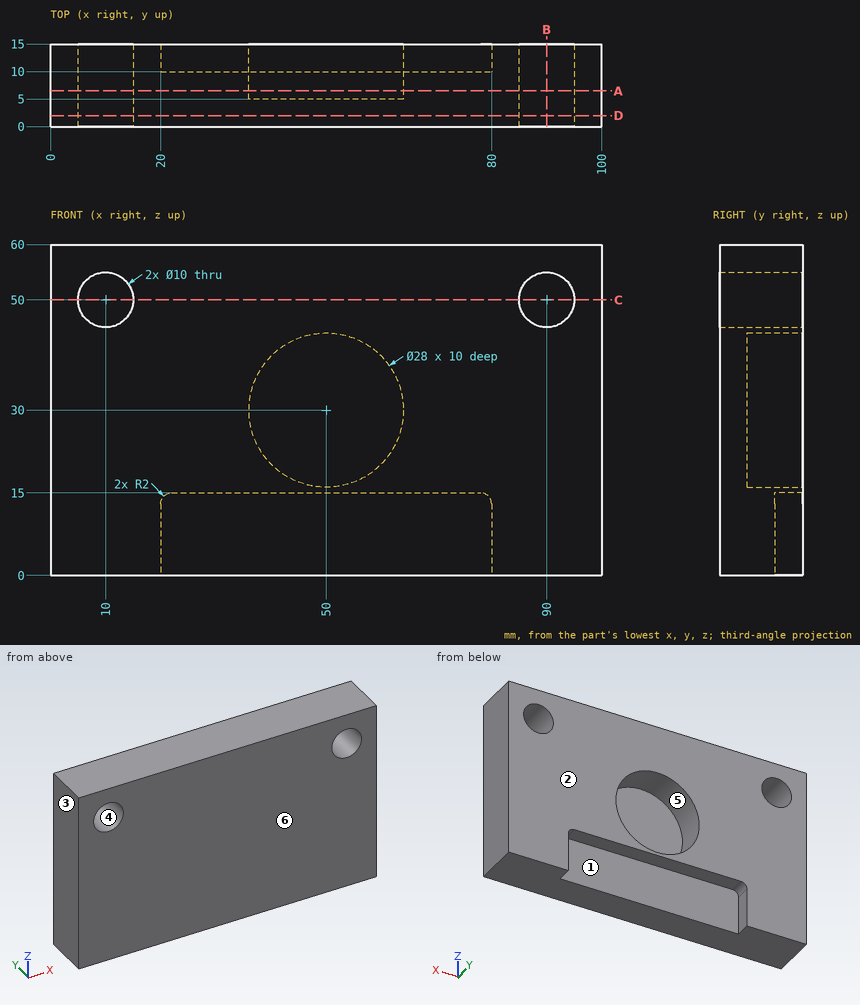
The drawing under review shows one solid part. Ordinate dimensions are in mm from its lowest x, y, z. A direction names the side the tool comes from. Coordinates: 2 decimals unless noted, no trailing zeros. Loops run counter-clockwise (first coordinate to the right, second up) from the corner with the lowest first, then second, coordinate; pieces in that order, holes last. Notation, with made-up numbers: (37, -39.75) -> (83, -39.75) arc R17 cw to (83, -26.75) -> close; hole circle Ø1 at (71.25, 81.25). An arc over 180 degrees is marked (long way). Answer as a JSON object with one key per item and string values.
Q1. Take a section at A-A on y = 6.5. Give the boundary of the cut face in (x, z), plus the area to 3 significant figures.
Answer block:
{"outline": "(0, 0) -> (100, 0) -> (100, 60) -> (0, 60) -> close; hole circle Ø10 at (10, 50); hole circle Ø28 at (50, 30); hole circle Ø10 at (90, 50)", "area": "5,230 mm^2"}
Q2. Take a section at D-D on y = 2. Give the boundary of the cut face in (x, z), plus the area to 3 significant figures.
Answer block:
{"outline": "(0, 0) -> (100, 0) -> (100, 60) -> (0, 60) -> close; hole circle Ø10 at (10, 50); hole circle Ø10 at (90, 50)", "area": "5,840 mm^2"}
Q3. Take a section at C-C on z = 50. Give the boundary of the cut face in (x, y).
Answer block:
{"outline": "(0, 0) -> (5, 0) -> (5, 15) -> (0, 15) -> close; (15, 0) -> (85, 0) -> (85, 15) -> (15, 15) -> close; (95, 0) -> (100, 0) -> (100, 15) -> (95, 15) -> close"}
Q4. Tool access review of the marked faces 5 and 6: name each direction out of +Z, -Z, +X, -X, +Y, -Y from which nothing blocks a thin tool from reaching the whole face with its end or side.
Answer block:
{"face 5": "+Y", "face 6": "+Z, -Z, +X, -X, -Y"}
Q5. Take a section at B-B on x = 90. Give the boundary of the cut face in (y, z), plus the area to 3 significant figures.
Answer block:
{"outline": "(0, 0) -> (15, 0) -> (15, 45) -> (0, 45) -> close; (0, 55) -> (15, 55) -> (15, 60) -> (0, 60) -> close", "area": "750 mm^2"}
Q6. Clearance check with flat-ended pins moving along their axes: pin 1 Ø7.5 at (x, z) = (40.5, 5.5) entering from +Y; pin 2 Ø4 at (x, y) = (51.5, 9) entering from -Z; pin 3 Ø1.5 at (x, y) = (41.5, 11.5) entering from -Z; pin 4 Ø8 at (x, z) = (10, 50) entering from +Y. State where each tip first meets the part, or that it passes through.
Answer block:
{"pin 1": "stops at y = 10", "pin 2": "stops at z = 0", "pin 3": "stops at z = 15", "pin 4": "passes through"}
Q7. The part is to be moulded in two halves that separate along X. For the marked faces 1, 2, 3 and 4, say which applies: +X half, -X half, draft (parallel to the pull), parting line (faces both ways), or undercut.
Answer block:
{"face 1": "undercut", "face 2": "draft", "face 3": "-X half", "face 4": "undercut"}
Q8. To check wall thickness, follow L1, parallel to X at y = 6, z = 50; L2, parallel to X at y = 13.25, z = 30; L3, parallel to Z at x = 10, y = 11.25. State the ranges of each line that lie inside material, in increasing order.
Answer block:
{"L1": "x = 0 to 5, 15 to 85, 95 to 100", "L2": "x = 0 to 36, 64 to 100", "L3": "z = 0 to 45, 55 to 60"}
